Input: part model. Units: mm. Frame: model coordinates. Coordinates: 2 decimals unless noted, no trailing zeros. Loops run counter-clockwise (first coordinate to the right, second up) from the corner with the lowest first, then second, coordinate; pieces in that order, holes last. Notation, with made-up numbers: M 66.5,55 L 111.5,55 A13 cw 111.5,78 Z; hole C -9,14 d8. An arc over 180 degrees is marked long. Use a Markdown table: item, result. Add a question column.
1. Pin query (flat end, axial travel): pin 1 (5 mm diameter, centred on x = -293, y = 206, fed in from +Z). Return the tip coordinate at first contact, or that it passes through.
2. Line query: L1, parallel to Y at x = -292.1, z = -5.5; L2, parallel to Y at x = 229, z = -11 (3 decimals); L3, parallel to Y at x = 66, z = -7.75 (3 decimals). Output: solid intervals per line, ascending. Write a range as [from, to].
3. Section A-A on y = 254. Output: boundary loops of the cut face in (x, z), then the cut area to 3 significant figures.
```python
from build123d import *

# Parameters (mm, degrees)
F0_W     = 609.6
F0_H     = 609.6
F0_R     = 7.540625
F0_R_2   = 5.159375
F1_DEPTH = 19.05
F2_DEPTH = 12.7
F3_W     = 609.6
F3_H     = 3.175
F4_DEPTH = 12.7
F5_W     = 25.4
F5_H     = 0.0254
F5_W_2   = 50
F6_DEPTH = 0.254
F8_DEPTH = 2.54


# Not quite as in the source:
# - a pattern or mirror of a feature is missing from the dataset's text; its kind, count and spacing are read off the source's solid
# - a feature names something its author has since deleted; it is built from what else it names


with BuildPart() as f1:
    # F0 (on Top) → F1 (new body)
    with BuildSketch(Plane.XY):
        Rectangle(F0_W, F0_H)
        with Locations((-271.4625, -269.875)):
            Circle(F0_R, mode=Mode.SUBTRACT)
        with Locations((-292.1, -220.6625)):
            Circle(F0_R_2, mode=Mode.SUBTRACT)
        with Locations((-292.1, -188.9125)):
            Circle(F0_R_2, mode=Mode.SUBTRACT)
        with Locations((-227.80625, -220.6625)):
            Circle(F0_R_2, mode=Mode.SUBTRACT)
        with Locations((-227.80625, -188.9125)):
            Circle(F0_R_2, mode=Mode.SUBTRACT)
        with Locations((-292.1, 206.375)):
            Circle(F0_R_2, mode=Mode.SUBTRACT)
        with Locations((-227.80625, 206.375)):
            Circle(F0_R_2, mode=Mode.SUBTRACT)
        with Locations((-292.1, 238.125)):
            Circle(F0_R_2, mode=Mode.SUBTRACT)
        with Locations((-271.4625, 254)):
            Circle(F0_R, mode=Mode.SUBTRACT)
        with Locations((-227.80625, 238.125)):
            Circle(F0_R_2, mode=Mode.SUBTRACT)
        with Locations((-227.80625, 206.375)):
            Circle(F0_R_2)
        with Locations((-227.80625, 238.125)):
            Circle(F0_R_2)
        with Locations((-227.80625, -188.9125)):
            Circle(F0_R_2)
        with Locations((-227.80625, -220.6625)):
            Circle(F0_R_2)
        with Locations((-271.4625, -269.875)):
            Circle(F0_R)
        with Locations((-271.4625, 254)):
            Circle(F0_R)
        with Locations((-292.1, 238.125)):
            Circle(F0_R_2)
        with Locations((-292.1, 206.375)):
            Circle(F0_R_2)
        with Locations((-292.1, -220.6625)):
            Circle(F0_R_2)
        with Locations((-292.1, -188.9125)):
            Circle(F0_R_2)
    extrude(amount=-F1_DEPTH)

    # F0 (on Top) → F2 (cut)
    with BuildSketch(Plane.XY):
        with Locations((-271.4625, -269.875)):
            Circle(F0_R)
        with Locations((-292.1, -220.6625)):
            Circle(F0_R_2)
        with Locations((-227.80625, -220.6625)):
            Circle(F0_R_2)
        with Locations((-227.80625, -188.9125)):
            Circle(F0_R_2)
        with Locations((-292.1, -188.9125)):
            Circle(F0_R_2)
        with Locations((-292.1, 206.375)):
            Circle(F0_R_2)
        with Locations((-227.80625, 206.375)):
            Circle(F0_R_2)
        with Locations((-227.80625, 238.125)):
            Circle(F0_R_2)
        with Locations((-292.1, 238.125)):
            Circle(F0_R_2)
        with Locations((-271.4625, 254)):
            Circle(F0_R)
    f2 = extrude(amount=-F2_DEPTH, mode=Mode.SUBTRACT)

    # F2_copies: F2 across plane
    add(f2.mirror(Plane(origin=(0, 0, 0), x_dir=(0, 0, 1), z_dir=(1, 0, 0))), mode=Mode.SUBTRACT)

    # F3 (on face) → F4 (cut)
    with BuildSketch(Plane(origin=(0, 0, -19.05), x_dir=(1, 0, 0), z_dir=(0, 0, -1))):
        with Locations((0, -293.6875)):
            Rectangle(F3_W, F3_H)
    extrude(amount=-F4_DEPTH, mode=Mode.SUBTRACT)

    # F5 (on face) → F6 (cut)
    with BuildSketch(Plane(origin=(0, 0, -19.05), x_dir=(1, 0, 0), z_dir=(0, 0, -1))):
        with Locations((-156.0546457767, -265.0721735465)):
            Rectangle(F5_W, F5_H)
        with Locations((-145.1898425817, -234.882380328)):
            Rectangle(F5_W_2, F5_H)
    extrude(amount=-F6_DEPTH, mode=Mode.SUBTRACT)

    # F7 (on face) → F8 (cut)
    with BuildSketch(Plane.XY):
        with BuildLine():
            Line((273.05, 304.8), (273.0246, 304.8))
            Line((273.0246, 304.8), (273.0246, 261.3770501544))
            ThreePointArc((273.0246, 261.3770501544), (273.0373023354, 261.3743489879), (273.05, 261.3716259496))
            Line((273.05, 261.3716259496), (273.05, 304.8))
        make_face()
        with BuildLine():
            ThreePointArc((273.05, 261.3716259496), (273.0373023354, 261.3743489879), (273.0246, 261.3770501544))
            Line((273.0246, 261.3770501544), (273.0246, 246.6229498456))
            ThreePointArc((273.0246, 246.6229498456), (273.0373023354, 246.6256510121), (273.05, 246.6283740504))
            Line((273.05, 246.6283740504), (273.05, 261.3716259496))
        make_face()
        with BuildLine():
            ThreePointArc((273.05, 246.6283740504), (273.0373023354, 246.6256510121), (273.0246, 246.6229498456))
            Line((273.0246, 246.6229498456), (273.0246, -262.4979498456))
            ThreePointArc((273.0246, -262.4979498456), (273.0373023354, -262.5006510121), (273.05, -262.5033740504))
            Line((273.05, -262.5033740504), (273.05, 246.6283740504))
        make_face()
        with BuildLine():
            ThreePointArc((273.05, -262.5033740504), (273.0373023354, -262.5006510121), (273.0246, -262.4979498456))
            Line((273.0246, -262.4979498456), (273.0246, -277.2520501544))
            ThreePointArc((273.0246, -277.2520501544), (273.0373023354, -277.2493489879), (273.05, -277.2466259496))
            Line((273.05, -277.2466259496), (273.05, -262.5033740504))
        make_face()
        with BuildLine():
            Line((273.0246, -277.2520501544), (273.0246, -304.8))
            Line((273.0246, -304.8), (273.05, -304.8))
            Line((273.05, -304.8), (273.05, -277.2466259496))
            ThreePointArc((273.05, -277.2466259496), (273.0373023354, -277.2493489879), (273.0246, -277.2520501544))
        make_face()
        with BuildLine():
            Line((-273.0246, 304.8), (-273.05, 304.8))
            Line((-273.05, 304.8), (-273.05, 261.3716259496))
            ThreePointArc((-273.05, 261.3716259496), (-273.0373023354, 261.3743489879), (-273.0246, 261.3770501544))
            Line((-273.0246, 261.3770501544), (-273.0246, 304.8))
        make_face()
        with BuildLine():
            ThreePointArc((-273.0246, 261.3770501544), (-273.0373023354, 261.3743489879), (-273.05, 261.3716259496))
            Line((-273.05, 261.3716259496), (-273.05, 246.6283740504))
            ThreePointArc((-273.05, 246.6283740504), (-273.0373023354, 246.6256510121), (-273.0246, 246.6229498456))
            Line((-273.0246, 246.6229498456), (-273.0246, 261.3770501544))
        make_face()
        with BuildLine():
            ThreePointArc((-273.0246, -262.4979498456), (-273.0373023354, -262.5006510121), (-273.05, -262.5033740504))
            Line((-273.05, -262.5033740504), (-273.05, -277.2466259496))
            ThreePointArc((-273.05, -277.2466259496), (-273.0373023354, -277.2493489879), (-273.0246, -277.2520501544))
            Line((-273.0246, -277.2520501544), (-273.0246, -262.4979498456))
        make_face()
        with BuildLine():
            Line((-273.05, -277.2466259496), (-273.05, -304.8))
            Line((-273.05, -304.8), (-273.0246, -304.8))
            Line((-273.0246, -304.8), (-273.0246, -277.2520501544))
            ThreePointArc((-273.0246, -277.2520501544), (-273.0373023354, -277.2493489879), (-273.05, -277.2466259496))
        make_face()
        with BuildLine():
            ThreePointArc((-273.0246, 246.6229498456), (-273.0373023354, 246.6256510121), (-273.05, 246.6283740504))
            Line((-273.05, 246.6283740504), (-273.05, -262.5033740504))
            ThreePointArc((-273.05, -262.5033740504), (-273.0373023354, -262.5006510121), (-273.0246, -262.4979498456))
            Line((-273.0246, -262.4979498456), (-273.0246, 246.6229498456))
        make_face()
    extrude(amount=-F8_DEPTH, mode=Mode.SUBTRACT)


solid = f1.part
```
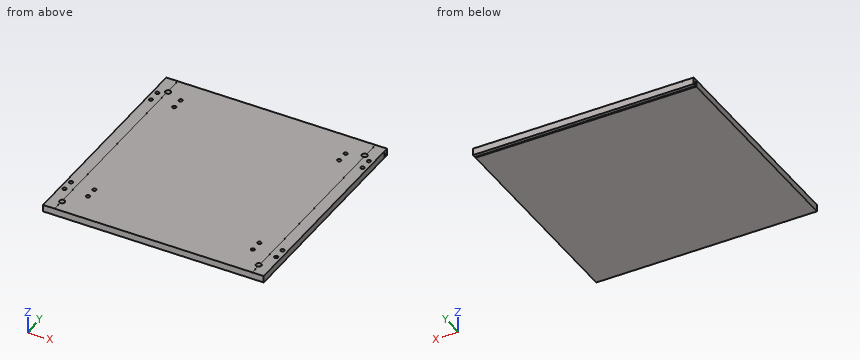
Answers below:
| question | item | result |
|---|---|---|
| 1 | pin 1 | stops at z = -12.7 |
| 2 | L1 | y = [-304.8, -225.82], [-215.5, -194.07], [-183.75, 201.22], [211.53, 232.97], [243.28, 304.8] |
| 2 | L2 | y = [-304.8, -225.682], [-215.643, -193.932], [-183.893, 201.356], [211.394, 233.106], [243.144, 292.1], [295.275, 304.8] |
| 2 | L3 | y = [-304.8, 292.1], [295.275, 304.8] |
| 3 | outline | M -304.8,-19.05 L 304.8,-19.05 L 304.8,0 L 279,0 L 279,-12.7 L 263.92,-12.7 L 263.92,0 L -263.92,0 L -263.92,-12.7 L -279,-12.7 L -279,0 L -304.8,0 Z |
| 3 | area | 11,200 mm² |
